Design review of the part built by this model. Coordinates are the model's own, in mm. A direction names the side the tool comes from. Give positions to 0.01 mm unless a question says otherwise; leave off trailing zeros. Loops run counter-clockwise (first coordinate to the right, second up) from the corner with the lowest first, then second, coordinate; pieces in that order, holes last. Notation, with made-up numbers: M 10.25,27.25 L 43.25,27.25 A21 ccw 43.25,61.25 Z; hole C -28,69.5 d4. An arc over 180 degrees is marked long. Use CSV: the item, a comma, the result in double quotes.
Autodesk Inventor part; units mm, degrees
ref_plane "YZ Plane" through (0, 0, 0) normal (1, 0, 0) x (0, 1, 0)
ref_plane "XZ Plane" through (0, 0, 0) normal (0, 1, 0) x (-1, 0, 0)
ref_plane "XY Plane" through (0, 0, 0) normal (0, 0, 1) x (1, 0, 0)
sketch "Sketch1" plane through (0, 0, 0) normal (0, 0, 1) x (1, 0, 0)
  line L0 (-14.2973, 4.3336) -> (-13.3453, 4.3336)
  line L1 (-18.3453, 6.2132) -> (6.6546, 6.2132)
  arc A0 (-14.971, 2.5331) -> (-14.5513, 3.9796) centre (-17.2541, 3.9796) ccw
  arc A1 (-17.1394, 3.9796) -> (-16.7197, 2.5331) centre (-14.4366, 3.9796) ccw
  arc A2 (-15.207, 2.4032) -> (-14.971, 2.5331) centre (-15.207, 2.6826) ccw
  arc A3 (-16.7197, 2.5331) -> (-16.4837, 2.4032) centre (-16.4837, 2.6826) ccw
  line L2 (-15.8453, 2.4032) -> (-15.207, 2.4032)
  line L3 (-15.8453, 2.4032) -> (-16.4837, 2.4032)
  arc A4 (-14.2973, 4.3336) -> (-14.5513, 4.0796) centre (-14.2973, 4.0796) ccw
  arc A5 (-17.1394, 4.0796) -> (-17.3934, 4.3336) centre (-17.3934, 4.0796) ccw
  line L4 (-18.3453, 4.3336) -> (-18.3453, 6.2132)
  line L5 (-14.5513, 3.9796) -> (-14.5513, 4.0796)
  line L6 (-17.3934, 4.3336) -> (-18.3453, 4.3336)
  line L7 (-17.1394, 3.9796) -> (-17.1394, 4.0796)
  arc A6 (5.029, 2.5331) -> (5.4487, 3.9796) centre (2.7459, 3.9796) ccw
  arc A7 (2.8606, 3.9796) -> (3.2803, 2.5331) centre (5.5634, 3.9796) ccw
  arc A8 (0.029, 2.5331) -> (0.4487, 3.9796) centre (-2.2541, 3.9796) ccw
  arc A9 (-2.1394, 3.9796) -> (-1.7197, 2.5331) centre (0.5634, 3.9796) ccw
  arc A10 (-4.971, 2.5331) -> (-4.5513, 3.9796) centre (-7.2541, 3.9796) ccw
  arc A11 (-7.1394, 3.9796) -> (-6.7197, 2.5331) centre (-4.4366, 3.9796) ccw
  arc A12 (-9.971, 2.5331) -> (-9.5513, 3.9796) centre (-12.2541, 3.9796) ccw
  arc A13 (-12.1394, 3.9796) -> (-11.7197, 2.5331) centre (-9.4366, 3.9796) ccw
  arc A14 (-10.207, 2.4032) -> (-9.971, 2.5331) centre (-10.207, 2.6826) ccw
  line L8 (-10.8453, 2.4032) -> (-10.207, 2.4032)
  arc A15 (-11.7197, 2.5331) -> (-11.4837, 2.4032) centre (-11.4837, 2.6826) ccw
  line L9 (-10.8453, 2.4032) -> (-11.4837, 2.4032)
  arc A16 (-5.207, 2.4032) -> (-4.971, 2.5331) centre (-5.207, 2.6826) ccw
  line L10 (-5.8453, 2.4032) -> (-5.207, 2.4032)
  arc A17 (-6.7197, 2.5331) -> (-6.4837, 2.4032) centre (-6.4837, 2.6826) ccw
  line L11 (-5.8453, 2.4032) -> (-6.4837, 2.4032)
  arc A18 (-0.207, 2.4032) -> (0.029, 2.5331) centre (-0.207, 2.6826) ccw
  line L12 (-0.8454, 2.4032) -> (-0.207, 2.4032)
  arc A19 (-1.7197, 2.5331) -> (-1.4837, 2.4032) centre (-1.4837, 2.6826) ccw
  line L13 (-0.8454, 2.4032) -> (-1.4837, 2.4032)
  arc A20 (4.793, 2.4032) -> (5.029, 2.5331) centre (4.793, 2.6826) ccw
  line L14 (4.1546, 2.4032) -> (4.793, 2.4032)
  arc A21 (3.2803, 2.5331) -> (3.5163, 2.4032) centre (3.5163, 2.6826) ccw
  line L15 (4.1546, 2.4032) -> (3.5163, 2.4032)
  line L16 (-2.3934, 4.3336) -> (-3.3454, 4.3336)
  line L17 (-9.2973, 4.3336) -> (-8.3453, 4.3336)
  line L18 (-9.5513, 3.9796) -> (-9.5513, 4.0796)
  arc A22 (-9.2973, 4.3336) -> (-9.5513, 4.0796) centre (-9.2973, 4.0796) ccw
  line L19 (-12.1394, 3.9796) -> (-12.1394, 4.0796)
  arc A23 (-12.1394, 4.0796) -> (-12.3934, 4.3336) centre (-12.3934, 4.0796) ccw
  line L20 (-12.3934, 4.3336) -> (-13.3453, 4.3336)
  line L21 (-4.5513, 3.9796) -> (-4.5513, 4.0796)
  arc A24 (-4.2973, 4.3336) -> (-4.5513, 4.0796) centre (-4.2973, 4.0796) ccw
  line L22 (-4.2973, 4.3336) -> (-3.3454, 4.3336)
  line L23 (-7.1394, 3.9796) -> (-7.1394, 4.0796)
  arc A25 (-7.1394, 4.0796) -> (-7.3934, 4.3336) centre (-7.3934, 4.0796) ccw
  line L24 (-7.3934, 4.3336) -> (-8.3453, 4.3336)
  line L25 (2.6066, 4.3336) -> (1.6546, 4.3336)
  line L26 (0.4487, 3.9796) -> (0.4487, 4.0796)
  arc A26 (0.7027, 4.3336) -> (0.4487, 4.0796) centre (0.7027, 4.0796) ccw
  line L27 (0.7027, 4.3336) -> (1.6546, 4.3336)
  line L28 (-2.1394, 3.9796) -> (-2.1394, 4.0796)
  arc A27 (-2.1394, 4.0796) -> (-2.3934, 4.3336) centre (-2.3934, 4.0796) ccw
  line L29 (5.4487, 3.9796) -> (5.4487, 4.0796)
  arc A28 (5.7027, 4.3336) -> (5.4487, 4.0796) centre (5.7027, 4.0796) ccw
  line L30 (5.7027, 4.3336) -> (6.6546, 4.3336)
  line L31 (2.8606, 3.9796) -> (2.8606, 4.0796)
  arc A29 (2.8606, 4.0796) -> (2.6066, 4.3336) centre (2.6066, 4.0796) ccw
  line L32 (6.6546, 4.3336) -> (6.6546, 6.2132)
  line L33 (6.0839, 4.3336) -> (6.6546, 4.3336)
  dimension "d2" = 5
  dimension "d3" = 3.81
  dimension "d4" = 1.9304
extrude "Extrusion1" add sketch "Sketch1" along normal blind 9
properties part number "5MR-535-09"
(1) We need section B-B on x = -8.25. State the section outline as (y, z) points.
A:
outline,"M 4.33,0 L 6.21,0 L 6.21,9 L 4.33,9 Z"
(2) Machinability: for faces 1 (the flat face through (-6, 5, 9)), 2 (the flat face through (6, 4.334, 4)), 3 (the cylindrical face through (-4.655, 3.237, 4.437)), which of the approach directions +Z, -Z, +X, -X, +Y, -Y give a long, thin tool a straight path to every point of the face, cutting with its end or side? Answer none if there is none.
A:
face 1,"+Z, +X, -X, +Y, -Y"
face 2,"+Z, -Z, +X, -Y"
face 3,"+Z, -Z, -Y"
(3) We need section A-A on y = 3.05. State the section outline as (x, z) points.
A:
outline,"M -16.97,0 L -14.72,0 L -14.72,9 L -16.97,9 Z; M -11.97,0 L -9.72,0 L -9.72,9 L -11.97,9 Z; M -6.97,0 L -4.72,0 L -4.72,9 L -6.97,9 Z; M -1.97,0 L 0.28,0 L 0.28,9 L -1.97,9 Z; M 3.03,0 L 5.28,0 L 5.28,9 L 3.03,9 Z"
(4) Clearance check with flat-ended pins moving along their axes: P1, Ø0.6, axis at x = -13.5, z = 6, coming from the -Y side; P2, Ø2, axis at y = 4, z = 6, coming from the -X side. State where each tip first meets the part, or that it passes through.
A:
P1,"y = 4.33"
P2,"x = -18.35"
(5) Wall thickness on line 1 along X through (y, z) = (4.1, 7); line 2 along X through (y, z) = (4.15, 3.75); line 3 along Y through (x, z) = (1.75, 1): over which ranges is each line inside the solid? List them lowest first. Write a range as [from, to].
A:
line 1,"[-17.14, -14.55], [-12.14, -9.55], [-7.14, -4.55], [-2.14, 0.45], [2.86, 5.45]"
line 2,"[-17.15, -14.54], [-12.15, -9.54], [-7.15, -4.54], [-2.15, 0.46], [2.85, 5.46]"
line 3,"[4.33, 6.21]"
